```python
from build123d import *

# Parameters (mm, degrees)
F0_W     = 0.64
F0_H     = 2.54
F1_DEPTH = 2.54
F2_DEPTH = 0.64


with BuildPart() as f1:
    # F0 (on Front) → F1 (new body)
    with BuildSketch(Plane.XZ):
        with BuildLine():
            Line((-0.32, 1.27), (-0.67, 1.27))
            ThreePointArc((-0.67, 1.27), (-1.0942640687, 1.0942640687), (-1.27, 0.67))
            Line((-1.27, 0.67), (-1.27, -0.67))
            ThreePointArc((-1.27, -0.67), (-1.0942640687, -1.0942640687), (-0.67, -1.27))
            Line((-0.67, -1.27), (-0.32, -1.27))
            Line((-0.32, -1.27), (-0.32, 1.27))
        make_face()
        with BuildLine():
            Line((0.67, 1.27), (0.32, 1.27))
            Line((0.32, 1.27), (0.32, -1.27))
            Line((0.32, -1.27), (0.67, -1.27))
            ThreePointArc((0.67, -1.27), (1.0942640687, -1.0942640687), (1.27, -0.67))
            Line((1.27, -0.67), (1.27, 0.67))
            ThreePointArc((1.27, 0.67), (1.0942640687, 1.0942640687), (0.67, 1.27))
        make_face()
        Rectangle(F0_W, F0_H)
    extrude(amount=F1_DEPTH)

    # F0 (on Front) → F2 (join)
    with BuildSketch(Plane.XZ):
        with BuildLine():
            Line((-0.32, 7.21), (-0.32, 1.27))
            Line((-0.32, 1.27), (0.32, 1.27))
            Line((0.32, 1.27), (0.32, 7.21))
            ThreePointArc((0.32, 7.21), (0.2614213562, 7.3514213562), (0.12, 7.41))
            Line((0.12, 7.41), (-0.12, 7.41))
            ThreePointArc((-0.12, 7.41), (-0.2614213562, 7.3514213562), (-0.32, 7.21))
        make_face()
        Rectangle(F0_W, F0_H)
        with BuildLine():
            Line((-0.32, 1.27), (-0.67, 1.27))
            ThreePointArc((-0.67, 1.27), (-1.0942640687, 1.0942640687), (-1.27, 0.67))
            Line((-1.27, 0.67), (-1.27, -0.67))
            ThreePointArc((-1.27, -0.67), (-1.0942640687, -1.0942640687), (-0.67, -1.27))
            Line((-0.67, -1.27), (-0.32, -1.27))
            Line((-0.32, -1.27), (-0.32, 1.27))
        make_face()
        with BuildLine():
            Line((0.67, 1.27), (0.32, 1.27))
            Line((0.32, 1.27), (0.32, -1.27))
            Line((0.32, -1.27), (0.67, -1.27))
            ThreePointArc((0.67, -1.27), (1.0942640687, -1.0942640687), (1.27, -0.67))
            Line((1.27, -0.67), (1.27, 0.67))
            ThreePointArc((1.27, 0.67), (1.0942640687, 1.0942640687), (0.67, 1.27))
        make_face()
        with BuildLine():
            Line((0.32, -1.27), (-0.32, -1.27))
            Line((-0.32, -1.27), (-0.32, -4.07))
            ThreePointArc((-0.32, -4.07), (-0.2614213562, -4.2114213562), (-0.12, -4.27))
            Line((-0.12, -4.27), (0.12, -4.27))
            ThreePointArc((0.12, -4.27), (0.2614213562, -4.2114213562), (0.32, -4.07))
            Line((0.32, -4.07), (0.32, -1.27))
        make_face()
    extrude(amount=F2_DEPTH)


solid = f1.part
```
Input: part model. Units: mm. Frame: model coordinates. Give positions to 0.01 mm unless a question says otherwise; leave off trailing zeros. Order: outer loops, then holes, each group sorted by start corner. A loop starts at its lowest first (then second) coordinate and runs counter-clockwise, first axis right, second up.
1. Section B-B on x = 0. Return the cut outline in (y, z), and give its area (3 significant figures).
Derived:
outline: (-2.54, -1.27) - (-0.64, -1.27) - (-0.64, -4.27) - (0, -4.27) - (0, 7.41) - (-0.64, 7.41) - (-0.64, 1.27) - (-2.54, 1.27) - close
area: 12.3 mm2
2. Section D-D on y = -0.35. Return the cut outline in (x, z), and give its area (3 significant figures).
Derived:
outline: (-1.27, -0.67) arc R0.6 ccw to (-0.67, -1.27) - (-0.32, -1.27) - (-0.32, -4.07) arc R0.2 ccw to (-0.12, -4.27) - (0.12, -4.27) arc R0.2 ccw to (0.32, -4.07) - (0.32, -1.27) - (0.67, -1.27) arc R0.6 ccw to (1.27, -0.67) - (1.27, 0.67) arc R0.6 ccw to (0.67, 1.27) - (0.32, 1.27) - (0.32, 7.21) arc R0.2 ccw to (0.12, 7.41) - (-0.12, 7.41) arc R0.2 ccw to (-0.32, 7.21) - (-0.32, 1.27) - (-0.67, 1.27) arc R0.6 ccw to (-1.27, 0.67) - close
area: 12.0 mm2
3. Section A-A on y = -1.95. Return the cut outline in (x, z).
Derived:
outline: (-1.27, -0.67) arc R0.6 ccw to (-0.67, -1.27) - (0.67, -1.27) arc R0.6 ccw to (1.27, -0.67) - (1.27, 0.67) arc R0.6 ccw to (0.67, 1.27) - (-0.67, 1.27) arc R0.6 ccw to (-1.27, 0.67) - close
4. Material intervals for L1, parallel to X at y = -0.25, z = 6; L2, parallel to Z at x = 0, y = -2.15; L3, parallel to Y at x = 0.15, z = 5.25, sorted ascending.
Derived:
L1: x = -0.32 to 0.32
L2: z = -1.27 to 1.27
L3: y = -0.64 to 0
5. Section C-C on z = 2.75. Return the cut outline in (x, y).
Derived:
outline: (-0.32, -0.64) - (0.32, -0.64) - (0.32, 0) - (-0.32, 0) - close
6. Pin query (flat end, axial travel): pin 1 (0.7 mm diameter, centred on x = 0, z = -2.5, fed in from -Y); pin 2 (0.7 mm diameter, centred on y = 0, z = 3.5, fed in from -X); pin 3 (1.5 mm diameter, centred on x = 0.5, z = 0.5, fed in from +Y). Return the tip coordinate at first contact, or that it passes through.
Derived:
pin 1: stops at y = -0.64
pin 2: stops at x = -0.32
pin 3: stops at y = 0
